from build123d import *

# Parameters (mm, degrees)
SKETCH_1_R      = 1.5
EXTRUDE_1_DEPTH = 44
SKETCH_2_R      = 11
EXTRUDE_2_DEPTH = 2
SKETCH_3_R      = 2.5
EXTRUDE_3_DEPTH = 26
SKETCH_4_W      = 16
SKETCH_4_H      = 6
EXTRUDE_4_DEPTH = 6


with BuildPart() as part:
    # 草图1 → 凸台-拉伸1 (new body)
    with BuildSketch(Plane.XY):
        Polygon((21, 0), (21, 16.6), (16.6, 21), (0, 21), (-16.6, 21), (-21, 16.6), (-21, 0), (-21, -16.6), (-16.6, -21), (0, -21), (16.6, -21), (21, -16.6), align=None)
        with Locations((15.5, 15.5)):
            Circle(SKETCH_1_R, mode=Mode.SUBTRACT)
        with Locations((15.5, -15.5)):
            Circle(SKETCH_1_R, mode=Mode.SUBTRACT)
        with Locations((-15.5, -15.5)):
            Circle(SKETCH_1_R, mode=Mode.SUBTRACT)
        with Locations((-15.5, 15.5)):
            Circle(SKETCH_1_R, mode=Mode.SUBTRACT)
    extrude(amount=EXTRUDE_1_DEPTH)

    # 草图2 → 凸台-拉伸2 (add)
    with BuildSketch(Plane.XY.offset(44)):
        Circle(SKETCH_2_R)
    extrude(amount=EXTRUDE_2_DEPTH)

    # 草图3 → 凸台-拉伸3 (add)
    with BuildSketch(Plane.XY.offset(44)):
        with Locations(Location((0, 0, 0), (0, 0, 180))):
            Circle(SKETCH_3_R)
    extrude(amount=EXTRUDE_3_DEPTH)

    # 草图4 → 凸台-拉伸4 (add)
    with BuildSketch(Plane(origin=(0, 21, 0), x_dir=(1, 0, 0), z_dir=(0, 1, 0))):
        with Locations((0, -6)):
            Rectangle(SKETCH_4_W, SKETCH_4_H)
    extrude(amount=EXTRUDE_4_DEPTH)


solid = part.part
CAD build for the part. Positions are in the model's coordinates, mm. A direction names the side the tool comes from. Coordinates: 2 decimals unless noted, no trailing zeros. Write each loop counter-clockwise with the first axis right and the second up, starting at its lowest first coordinate (ties: lowest second). Pieces come first, ordered by that corner, then holes. Notation, with made-up numbers: M 29.5,37 L 65.5,37 A32 ccw 65.5,74 Z; hole C -38,69.5 d1. An arc over 180 degrees is marked long. Answer as a JSON object with one key per item and string values. Group by question number.
1) Mould opens along Y. For faces 1 (the face through (0, -21, 22)), 2 (the face through (-2.38, -10.74, 44.99)), 3 (the face through (-17, 15.57, 21.69)), 4 (the face through (21, 0, 22)) say: +Y half, -Y half, draft (parallel to the pull), parting line (faces both ways), or undercut.
2) Pin check, flat tips, straight feed: pin 1 Ø1.8 at (x, y) = (-2, 24) entering from -Z; pin 2 Ø1 at (y, z) = (18.5, 15.5) entering from -X; pin 3 Ø5 at (y, z) = (23, 6.5) entering from -X; pin 4 Ø2.5 at (x, y) = (-15.5, 15.5) entering from +Z. Stop position of each tip, or through.
3) Saw through at D-D (y = -4). Write the cut outline in (x, z).
4) Tool access for faces 5 (the face through (9, -9, 44)), 6 (the face through (0, 24, 9)), 7 (the face through (8, 24, 6)), 8 (the face through (-8, 24, 6)): list every direction of +Z, -Z, +X, -X, +Y, -Y with a clear straight run to the whole face (end or side of a thin tool).
5) Saw through at C-C (x = 0). Write the cut outline in (y, z), plus the area to 3 significant figures.
6) Wall check: line 1 (Y direction, x = 15.5, z = 16.5); line 2 (X direction, y = -16.5, z = 30.5); line 3 (Y direction, x = 15, z = 22). Give the ranges that are in metal, low to high. Write a range as from..to.
7) Saw through at A-A (x = 15.5). Write the cut outline in (y, z), plus the area to 3 significant figures.
Values follow:
{
 "1": {"face 1": "-Y half", "face 2": "parting line", "face 3": "undercut", "face 4": "draft"},
 "2": {"pin 1": "stops at z = 3", "pin 2": "stops at x = -19.6", "pin 3": "stops at x = -17.1", "pin 4": "passes through"},
 "3": {"outline": "M -21,0 L 21,0 L 21,44 L 10.25,44 L 10.25,46 L -10.25,46 L -10.25,44 L -21,44 Z"},
 "4": {"face 5": "+Z", "face 6": "+Z, +X, -X, +Y", "face 7": "+Z, -Z, +X, +Y", "face 8": "+Z, -Z, -X, +Y"},
 "5": {"outline": "M -21,0 L 21,0 L 21,3 L 27,3 L 27,9 L 21,9 L 21,44 L 11,44 L 11,46 L 2.5,46 L 2.5,70 L -2.5,70 L -2.5,46 L -11,46 L -11,44 L -21,44 Z", "area": "2,050 mm2"},
 "6": {"line 1": "y = -21..-17, -14..14, 17..21", "line 2": "x = -21..-16.62, -14.38..14.38, 16.62..21", "line 3": "y = -21..-16.91, -14.09..14.09, 16.91..21"},
 "7": {"outline": "M -21,0 L -17,0 L -17,44 L -21,44 Z; M -14,0 L 14,0 L 14,44 L -14,44 Z; M 17,0 L 21,0 L 21,44 L 17,44 Z", "area": "1,580 mm2"}
}
